Autodesk Inventor part; units mm, degrees
ref_plane "YZ Plane" through (0, 0, 0) normal (1, 0, 0) x (0, 1, 0)
ref_plane "XZ Plane" through (0, 0, 0) normal (0, 1, 0) x (-1, 0, 0)
ref_plane "XY Plane" through (0, 0, 0) normal (0, 0, 1) x (1, 0, 0)
sketch "Sketch1" plane through (0, 0, 0) normal (1, 0, 0) x (0, 1, 0)
  line L0 (0, 0) -> (38.1, 0)
  line L1 (38.1, 0) -> (38.1, -101.6)
  line L2 (38.1, -101.6) -> (0, -101.6)
  line L3 (0, -101.6) -> (0, 0)
  dimension "d0" = 101.6
  dimension "d1" = 38.1
extrude "Extrusion1" add sketch "Sketch1" along normal blind 6.35
sketch "Sketch2" plane through (0, 0, 0) normal (-1, 0, 0) x (0, 0, 1)
  line L0 (0, 0) -> (0, 38.1)
  line L1 (-101.6, 38.1) -> (-101.6, 0)
  line L2 (-101.6, 0) -> (0, 0)
  line L3 (0, 0) -> (-101.6, 0)
  line L4 (-78.74, 0) -> (-74.295, 0)
  line L5 (-74.295, 0) -> (-74.295, 20.32)
  line L6 (-74.295, 20.32) -> (-78.74, 20.32)
  line L7 (-78.74, 20.32) -> (-78.74, 0)
  line L8 (-27.305, 0) -> (-22.86, 0)
  line L9 (-22.86, 0) -> (-22.86, 20.32)
  line L10 (-22.86, 20.32) -> (-27.305, 20.32)
  line L11 (-27.305, 20.32) -> (-27.305, 0)
  dimension "d10" = 4.445
  dimension "d11" = 4.445
  dimension "d13" = 20.32
  dimension "d14" = 22.86
  dimension "d15" = 22.86
extrude "Extrusion2" add sketch "Sketch2" along normal blind 19.05
chamfer "Chamfer1" distance 16.51 angle 45 2 edges at (-19.05, 20.32, -25.0825) (-19.05, 20.32, -76.5175)
sketch "Sketch3" plane through (0, 0, -101.6) normal (0, -1, 0) x (1, 0, 0)
  line L0 (0, 0) -> (6.35, 0)
  line L1 (9.525, -3.175) -> (-22.225, -3.175)
  line L2 (0, 101.6) -> (6.35, 101.6)
  line L3 (9.525, -3.175) -> (9.525, 104.775)
  line L4 (9.525, 104.775) -> (-22.225, 104.775)
  line L5 (-22.225, -3.175) -> (-22.225, 104.775)
  line L6 (-19.05, 22.86) -> (-19.05, 27.305)
  line L7 (6.35, 101.6) -> (6.35, 0)
  dimension "d22" = 3.175
  dimension "d25" = 3.175
  dimension "d26" = 3.175
  dimension "d27" = 3.175
  dimension "d52" = 107.95
  dimension "d53" = 31.75
extrude "Extrusion3" add sketch "Sketch3" along normal blind 6.35
sketch "Sketch4" plane through (0, 0, -101.6) normal (0, 1, 0) x (1, 0, 0)
  line L0 (0, -101.6) -> (6.35, -101.6)
  line L1 (0, -101.6) -> (6.35, -101.6)
  line L2 (6.35, -101.6) -> (6.35, 0)
  line L3 (6.35, -101.6) -> (6.35, 0)
  line L4 (6.35, 0) -> (0, 0)
  line L5 (0, 0) -> (0, 3.175)
  line L6 (9.525, 3.175) -> (-22.225, 3.175)
  line L7 (0, 3.175) -> (9.525, 3.175)
  line L8 (9.525, 3.175) -> (9.525, -104.775)
  line L9 (9.525, 3.175) -> (9.525, -104.775)
  line L10 (9.525, -104.775) -> (0, -104.775)
  line L11 (-22.225, -104.775) -> (9.525, -104.775)
  line L12 (0, -104.775) -> (0, -101.6)
extrude "Extrusion5" add sketch "Sketch4" along normal blind 6.35
sketch "Sketch5" plane through (0, 38.1, 0) normal (0, 1, 0) x (1, 0, 0)
  line L0 (0, 0) -> (0, -3.175)
  line L1 (0, 0) -> (6.35, 0)
  line L2 (6.35, 0) -> (6.35, 101.6)
  line L3 (6.35, 101.6) -> (0, 101.6)
  line L4 (0, 101.6) -> (0, 0)
extrude "Extrusion6" cut sketch "Sketch5" against normal blind 38.1
properties part number "MonsterHolder"
Could you check a few things on this model? Use its own coordinates, in mm. A direction names the side the tool comes from. Coordinates: 2 decimals unless noted, no trailing zeros. Order: outer loops, then holes, each group sorted by start corner. A loop starts at its lowest first (then second) coordinate and runs counter-clockwise, first axis right, second up. Notation, with made-up numbers: (36, -2.75) -> (56, -2.75) arc R22 ccw to (56, 6.25) -> close; hole circle Ø1 at (30.5, 34.5). An arc over 180 degrees is marked (long way). One line per item, written item: value. Start each with the question number.
1) If I drill on L1, parallel to Z at x = -9, y = 6.25 (3 decimals); L2, parallel to X at y = 1.25, z = -24 (3 decimals); L3, parallel to Y at x = 0, z = -80, over which ranges is the centre line in solid material (lowest first)? Write a range as [from, to].
2) Imagine slicing it at A-A on y = 15.25. List the corners of the cut face in (x, z) for me (3 decimals).
3) I'm going to push flat-ended pins straight in: pin 1 (1.1 mm diameter, centred on y = 2, z = -25, fed in from -X); pin 2 (6 mm diameter, centred on x = -12.5, z = -31, fed in from +Y); pin 3 (15 mm diameter, centred on x = -9.5, y = 7, fed in from +Z) (3 decimals); pin 4 (4 mm diameter, centred on x = -5.5, y = 17.5, fed in from -Z). Where does each tip first touch, or does it pass through?
4) Imagine slicing it at D-D on z = -63.5. List the corners of the cut face in (x, y) for me (3 decimals), plus the area to 3 significant figures.
5) Which directions (+Z, -Z, +X, -X, +Y, -Y) give clear straight access to the entire face, cutting with the end or side of a thin tool? Please do faces 4 (the flat face through (-3, -2, -104.775)), 5 (the flat face through (-19.05, 2, -77)), 6 (the flat face through (-7, 8, -27.305)), 7 (the flat face through (-7, 8, -22.86)), 8 (the flat face through (9.525, 0, -52)).
6) Imagine slicing it at C-C on x = 1.5. List the corners of the cut face in (y, z) for me (3 decimals), plus the area to 3 significant figures.
7) We'd pull the mould along X, two halves only. Please class faces 1 (the flat face through (-10.91, 11.95, -25.11)), 2 (the flat face through (3, 3, -101.6)), 3 (the flat face through (0, 10, -25)): +X half, -X half, draft (parallel to the pull), parting line (faces both ways), or undercut.
8) Imagine slicing it at B-B on y = 4.75. List the corners of the cut face in (x, z) for me (3 decimals).
Answer list:
1. L1: z = [-78.74, -74.295], [-27.305, -22.86]
1. L2: x = [-19.05, 0], [6.35, 9.525]
1. L3: y = [-6.35, 0]
2. outline: (-7.61, -78.74) -> (0, -78.74) -> (0, -74.295) -> (-7.61, -74.295) -> close; (-7.61, -27.305) -> (0, -27.305) -> (0, -22.86) -> (-7.61, -22.86) -> close
3. pin 1: stops at x = -19.05
3. pin 2: stops at y = 0
3. pin 3: stops at z = 3.175
3. pin 4: stops at z = -78.74
4. outline: (-22.225, -6.35) -> (9.525, -6.35) -> (9.525, 6.35) -> (6.35, 6.35) -> (6.35, 0) -> (-22.225, 0) -> close
4. area: 222 mm2
5. face 4: -Z, +X, -X, +Y, -Y
5. face 5: +Z, -Z, -X, +Y
5. face 6: -X, +Y
5. face 7: +Z, -X, +Y
5. face 8: +Z, -Z, +X, +Y, -Y
6. outline: (-6.35, -104.775) -> (6.35, -104.775) -> (6.35, -101.6) -> (0, -101.6) -> (0, 0) -> (6.35, 0) -> (6.35, 3.175) -> (-6.35, 3.175) -> close
6. area: 726 mm2
7. face 1: -X half
7. face 2: draft
7. face 3: undercut
8. outline: (-18.11, -78.74) -> (0, -78.74) -> (0, -74.295) -> (-18.11, -74.295) -> close; (-18.11, -27.305) -> (0, -27.305) -> (0, -22.86) -> (-18.11, -22.86) -> close; (0, -104.775) -> (9.525, -104.775) -> (9.525, 3.175) -> (0, 3.175) -> (0, 0) -> (6.35, 0) -> (6.35, -101.6) -> (0, -101.6) -> close
